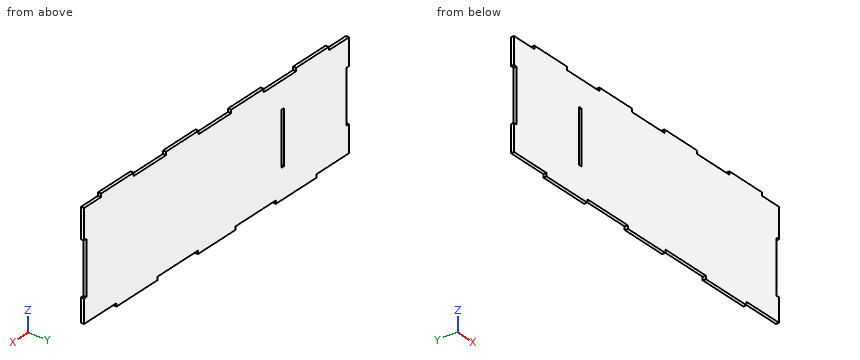
```python
from build123d import *

# Parameters (mm, degrees)
SKETCH1_W           = 326
SKETCH1_H           = 3
BOSS_EXTRUDE1_DEPTH = 100
SKETCH2_W           = 50
SKETCH2_H           = 3
SKETCH2_W_2         = 46
BOSS_EXTRUDE2_DEPTH = 3
SKETCH3_W           = 3
SKETCH3_H           = 50
CUT_EXTRUDE1_DEPTH  = 6
SKETCH4_W           = 3
SKETCH4_H           = 50
CUT_EXTRUDE2_DEPTH  = 6
SKETCH5_W           = 3
SKETCH5_H           = 50
CUT_EXTRUDE3_DEPTH  = 6
SKETCH6_W           = 40
SKETCH6_H           = 3
BOSS_EXTRUDE3_DEPTH = 3


with BuildPart() as part:
    # Sketch1 → Boss-Extrude1 (new body)
    with BuildSketch(Plane.XY):
        with Locations((0, -1.5)):
            Rectangle(SKETCH1_W, SKETCH1_H)
    extrude(amount=BOSS_EXTRUDE1_DEPTH)

    # Sketch2 → Boss-Extrude2 (add)
    with BuildSketch(Plane(origin=(0, 0, 0), x_dir=(-1, 0, 0), z_dir=(0, 0, -1))):
        with Locations((-98, -1.5)):
            Rectangle(SKETCH2_W, SKETCH2_H)
        with Locations((0, -1.5)):
            Rectangle(SKETCH2_W_2, SKETCH2_H)
        with Locations((98, -1.5)):
            Rectangle(SKETCH2_W, SKETCH2_H)
    extrude(amount=BOSS_EXTRUDE2_DEPTH)

    # Sketch3 → Cut-Extrude1 (cut)
    with BuildSketch(Plane.XZ.offset(3)):
        with Locations((-161.5, 50)):
            Rectangle(SKETCH3_W, SKETCH3_H)
    extrude(amount=-CUT_EXTRUDE1_DEPTH, mode=Mode.SUBTRACT)

    # Sketch4 → Cut-Extrude2 (cut)
    with BuildSketch(Plane.XZ.offset(3)):
        with Locations((-81.5, 50)):
            Rectangle(SKETCH4_W, SKETCH4_H)
    extrude(amount=-CUT_EXTRUDE2_DEPTH, mode=Mode.SUBTRACT)

    # Sketch5 → Cut-Extrude3 (cut)
    with BuildSketch(Plane.XZ.offset(3)):
        with Locations((161.5, 47)):
            Rectangle(SKETCH5_W, SKETCH5_H)
    extrude(amount=-CUT_EXTRUDE3_DEPTH, mode=Mode.SUBTRACT)

    # Sketch6 → Boss-Extrude3 (add)
    with BuildSketch(Plane.XY.offset(100)):
        with Locations((-118, -1.5)):
            Rectangle(SKETCH6_W, SKETCH6_H)
        with Locations((-38, -1.5)):
            Rectangle(SKETCH6_W, SKETCH6_H)
        with Locations((42, -1.5)):
            Rectangle(SKETCH6_W, SKETCH6_H)
        with Locations((122, -1.5)):
            Rectangle(SKETCH6_W, SKETCH6_H)
    extrude(amount=BOSS_EXTRUDE3_DEPTH)


solid = part.part
```
CAD build for the part. Positions are in the model's coordinates, mm. Coordinates: 2 decimals unless noted, no trailing zeros. Order: outer loops, then holes, each group sorted by start corner. A loop starts at its lowest first (then second) coordinate and runs counter-clockwise, first axis right, second up.
(1) Saw through at B-B, the plane x = 5.5. Write the cut outline in (y, z).
Solution:
outline: (-3, -3) - (0, -3) - (0, 100) - (-3, 100) - close
(2) Saw through at A-A, the plane z = 63.5. Write the cut outline in (x, y).
Solution:
outline: (-160, -3) - (-83, -3) - (-83, 0) - (-160, 0) - close; (-80, -3) - (160, -3) - (160, 0) - (-80, 0) - close
(3) Pin check, flat tips, straight feed: pin 1 Ø1.5 at (x, y) = (161.5, -1.5) entering from +Z; pin 2 Ø0.9 at (y, z) = (-1, 55.5) entering from -X; pin 3 Ø1.5 at (y, z) = (-2, -1) entering from +X. Stop position of each tip, or through.
Solution:
pin 1: stops at z = 100
pin 2: stops at x = -160
pin 3: stops at x = 123
(4) Drill centre lines: L1, parallel to X at y = -2.85, z = 45; L2, parallel to Z at x = -97, y = -0.7; L3, parallel to Z at x = 53, y = -0.2. Where is each one in solid material? Low to high.
Solution:
L1: x = -160 to -83, -80 to 160
L2: z = -3 to 100
L3: z = 0 to 103
